The listing builds one solid part. Answer for the finished solid, in the listing's coordinates (mm). Face numbers are marked on the shaded views. A direction names the side the tool comes from. Give positions to 0.01 mm unless a question says otherwise; leave off trailing zeros. Write each loop counter-clockwise with the first axis right and the second up, starting at its lowest first coordinate (ties: lowest second). Pieces come first, ordered by that corner, then holes. Notation, with made-up numbers: M 25.25,89.25 L 62.25,89.25 A33 cw 62.25,121.25 Z; hole C 67.5,11 d11. An arc over 180 degrees is marked long. Return JSON: item names as keys, results as strings.
from build123d import *

# Parameters (mm, degrees)
BOSS_EXTRUDE1_DEPTH   = 1.6
SKETCH2_R             = 3.45
BOSS_EXTRUDE2_DEPTH   = 1.4
M5X0_8_TAPPED_HOLE1_D = 3.2


with BuildPart() as part:
    # Sketch1 → Boss-Extrude1 (new body)
    with BuildSketch(Plane.XY):
        with BuildLine():
            Line((-6.237396753, 4.481095129), (-3, 5))
            Line((-3, 5), (3, 5))
            Line((3, 5), (6.237396753, 4.481095129))
            ThreePointArc((6.237396753, 4.481095129), (7.141511088, 3.973114811), (7.5, 3))
            Line((7.5, 3), (7.5, -3))
            ThreePointArc((7.5, -3), (7.141511088, -3.973114811), (6.237396753, -4.481095129))
            Line((6.237396753, -4.481095129), (3, -5))
            Line((3, -5), (-3, -5))
            Line((-3, -5), (-6.237396753, -4.481095129))
            ThreePointArc((-6.237396753, -4.481095129), (-7.141511088, -3.973114811), (-7.5, -3))
            Line((-7.5, -3), (-7.5, 3))
            ThreePointArc((-7.5, 3), (-7.141511088, 3.973114811), (-6.237396753, 4.481095129))
        make_face()
    extrude(amount=BOSS_EXTRUDE1_DEPTH)

    # Sketch2 → Boss-Extrude2 (add)
    with BuildSketch(Plane.XY.offset(1.6)):
        Circle(SKETCH2_R)
    extrude(amount=BOSS_EXTRUDE2_DEPTH)

    # M5x0.8 Tapped Hole1 (through all)
    with Locations(Plane.XY.offset(3)):
        with Locations((0, 0)):
            Hole(M5X0_8_TAPPED_HOLE1_D / 2)


solid = part.part
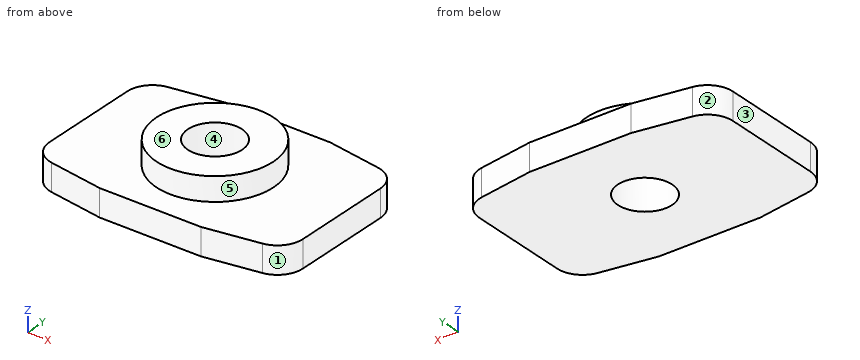
Item 1: A cutting plane is placed at A-A, the plane z = 0.5. Write down the section's boundary in (x, y).
Geometry results:
{"outline": "M -7.5,-3 A1.5 ccw -6.24,-4.48 L -3,-5 L 3,-5 L 6.24,-4.48 A1.5 ccw 7.5,-3 L 7.5,3 A1.5 ccw 6.24,4.48 L 3,5 L -3,5 L -6.24,4.48 A1.5 ccw -7.5,3 Z; hole C 0,0 d3.2"}
Item 2: Determine the mould class of the marked faces 1, 2, 3 and 4 for opening direction Y: +Y half, -Y half, draft (parallel to the pull), parting line (faces both ways), or undercut.
Geometry results:
{"face 1": "-Y half", "face 2": "+Y half", "face 3": "draft", "face 4": "undercut"}
Item 3: Which of the six approach directions +Z, -Z, +X, -X, +Y, -Y give full straight-line access (tool end or side, diameter ignored) to the marked faces 5 and 6?
Geometry results:
{"face 5": "+Z", "face 6": "+Z, +X, -X, +Y, -Y"}
Item 4: A cutting plane is placed at C-C, the plane y = 0.25. Write down the section's boundary in (x, z).
Geometry results:
{"outline": "M -7.5,0 L -1.58,0 L -1.58,3 L -3.44,3 L -3.44,1.6 L -7.5,1.6 Z; M 1.58,0 L 7.5,0 L 7.5,1.6 L 3.44,1.6 L 3.44,3 L 1.58,3 Z"}
Item 5: A cutting plane is placed at D-D, the plane x = 1.75. Write down the section's boundary in (y, z), plus the area to 3 significant figures.
Geometry results:
{"outline": "M -5,0 L 5,0 L 5,1.6 L 2.97,1.6 L 2.97,3 L -2.97,3 L -2.97,1.6 L -5,1.6 Z", "area": "24.3 mm2"}
Item 6: A cutting plane is placed at B-B, the plane x = -1.25. Write down the section's boundary in (y, z), plus the area to 3 significant figures.
Geometry results:
{"outline": "M -5,0 L -1,0 L -1,3 L -3.22,3 L -3.22,1.6 L -5,1.6 Z; M 1,0 L 5,0 L 5,1.6 L 3.22,1.6 L 3.22,3 L 1,3 Z", "area": "19.0 mm2"}
Item 7: Find the intervals of material crossed by line 1 (Y direction, x = 0, z = 0.9); line 2 (Y direction, x = 0, z = 2.3); line 3 (Z direction, x = -1, y = -4.25), in increasing order.
Geometry results:
{"line 1": "y = -5 to -1.6, 1.6 to 5", "line 2": "y = -3.45 to -1.6, 1.6 to 3.45", "line 3": "z = 0 to 1.6"}
